```python
from build123d import *

# Parameters (mm, degrees)
SKETCH1_W           = 63
SKETCH1_H           = 22
SKETCH1_R           = 1.15
BOSS_EXTRUDE1_DEPTH = 19
SKETCH2_R           = 2.65
BOSS_EXTRUDE2_DEPTH = 8


with BuildPart() as part:
    # Sketch1 → Boss-Extrude1 (new body)
    with BuildSketch(Plane.XY):
        with Locations((31.5, 11)):
            Rectangle(SKETCH1_W, SKETCH1_H)
        with Locations((32, 19.5)):
            Circle(SKETCH1_R, mode=Mode.SUBTRACT)
        with Locations((32, 2.5)):
            Circle(SKETCH1_R, mode=Mode.SUBTRACT)
    extrude(amount=BOSS_EXTRUDE1_DEPTH)

    # Sketch2 → Boss-Extrude2 (add)
    with BuildSketch(Plane.XY.offset(19)):
        with Locations(Location((52, 11, 0), (0, 0, 180))):
            Circle(SKETCH2_R)
    extrude(amount=BOSS_EXTRUDE2_DEPTH)


solid = part.part
```
Check sheet for the modelled part. Datum: model origin and axes. Units: mm. Give positions to 0.01 mm unless a question says otherwise; leave off trailing zeros. Order: outer loops, then holes, each group sorted by start corner. A loop starts at its lowest first (then second) coordinate and runs counter-clockwise, first axis right, second up. Notation, with made-up numbers: M 11,-4.5 L 32,-4.5 A20 cw 32,3.5 Z; hole C 45.25,27 d6. An arc over 180 degrees is marked long. Answer in a Markdown table with one row per item. Add a question column.
Q1. Release check for a two-part mould opening along X. For faces 1 (the cylindrical face through (32.53, 18.48, 9.37)), 2 (the cylindrical face through (49.55, 12.01, 22.94)), 3 (the cylindrical face through (33.062, 2.06, 9.367)), 4 (the flat face through (31, 11, 19)) record: released by +X, released by -X, zero draft, split by the parting line, or undercut.
Q2. Gauge pin test, flat ends, axial feed: pin 1 Ø10 at (y, z) = (4, 10.5) entering from -X; pin 2 Ø4 at (x, y) = (40, 16) entering from +Z; pin 3 Ø1.8 at (x, y) = (32, 19.5) entering from -Z. Record the tip position at first contact, or that the pin passes through.
Q3. Sectioned sample at A-A, the plane y = 19.5. Record the boundary of the cut face in (x, z), and give its area (3 significant figures).
Q4. Sectioned sample at C-C, the plane x = 30. Record the boundary of the cut face in (y, z), and give its area (3 significant figures).
Q5. Sectioned sample at B-B, the plane y = 11. Record the boundary of the cut face in (x, z), and give its area (3 significant figures).
Q6. Sectioned sample at D-D, the plane y = 5.25. Record the boundary of the cut face in (x, z), and give its area (3 significant figures).
Q7. Thickness scan on L1, parallel to Y at x = 32, z = 4.75; L2, parallel to Z at x = 53.5, y = 5.25; L3, parallel to X at y = 3, z = 14. Record the ranges inside material, lowest first.
Verdict:
| question | item | result |
|---|---|---|
| 1 | face 1 | undercut |
| 1 | face 2 | split by the parting line |
| 1 | face 3 | undercut |
| 1 | face 4 | zero draft |
| 2 | pin 1 | x = 0 |
| 2 | pin 2 | z = 19 |
| 2 | pin 3 | through |
| 3 | outline | M 0,0 L 30.85,0 L 30.85,19 L 0,19 Z; M 33.15,0 L 63,0 L 63,19 L 33.15,19 Z |
| 3 | area | 1,150 mm² |
| 4 | outline | M 0,0 L 22,0 L 22,19 L 0,19 Z |
| 4 | area | 418 mm² |
| 5 | outline | M 0,0 L 63,0 L 63,19 L 54.65,19 L 54.65,27 L 49.35,27 L 49.35,19 L 0,19 Z |
| 5 | area | 1,240 mm² |
| 6 | outline | M 0,0 L 63,0 L 63,19 L 0,19 Z |
| 6 | area | 1,200 mm² |
| 7 | L1 | 0 to 1.35, 3.65 to 18.35, 20.65 to 22 |
| 7 | L2 | 0 to 19 |
| 7 | L3 | 0 to 30.96, 33.04 to 63 |
